```python
from build123d import *

# Parameters (mm, degrees)
SKETCH1_R           = 15
BOSS_EXTRUDE5_DEPTH = 40
SKETCH1_12_R        = 5
BOSS_EXTRUDE6_DEPTH = 8
SKETCH2_W           = 12
SKETCH2_H           = 18
CUT_EXTRUDE1_DEPTH  = 68


with BuildPart() as part:
    # Sketch1 → Boss-Extrude5 (new body)
    with BuildSketch(Plane.XY):
        with BuildLine():
            ThreePointArc((22.912878475, 10), (25, 0), (22.912878475, -10))
            ThreePointArc((22.912878475, -10), (0, -25), (-22.912878475, -10))
            ThreePointArc((-22.912878475, -10), (-25, 0), (-22.912878475, 10))
            ThreePointArc((-22.912878475, 10), (0, 25), (22.912878475, 10))
        make_face()
        Circle(SKETCH1_R, mode=Mode.SUBTRACT)
    extrude(amount=BOSS_EXTRUDE5_DEPTH)

    # Sketch1_12 → Boss-Extrude6 (add)
    with BuildSketch(Plane.XY):
        with BuildLine():
            Line((35, 10), (22.912878475, 10))
            ThreePointArc((22.912878475, 10), (25, 0), (22.912878475, -10))
            Line((22.912878475, -10), (35, -10))
            ThreePointArc((35, -10), (45, 0), (35, 10))
        make_face()
        with Locations((35, 0)):
            Circle(SKETCH1_12_R, mode=Mode.SUBTRACT)
        with BuildLine():
            ThreePointArc((-22.912878475, 10), (-25, 0), (-22.912878475, -10))
            Line((-22.912878475, -10), (-35, -10))
            ThreePointArc((-35, -10), (-45, 0), (-35, 10))
            Line((-35, 10), (-22.912878475, 10))
        make_face()
        with Locations((-35, 0)):
            Circle(SKETCH1_12_R, mode=Mode.SUBTRACT)
    extrude(amount=BOSS_EXTRUDE6_DEPTH)

    # Sketch2 → Cut-Extrude1 (cut)
    with BuildSketch(Plane(origin=(25, 0, 0), x_dir=(0, 0, -1), z_dir=(1, 0, 0))):
        with Locations((-34, 0)):
            Rectangle(SKETCH2_W, SKETCH2_H)
    extrude(amount=-CUT_EXTRUDE1_DEPTH, mode=Mode.SUBTRACT)


solid = part.part
```
Geometry: final body of the model. Coordinates: model frame, mm. A direction names the side the tool comes from. Round coordinates to 2 decimals unless told otherwise and drop trailing zeros. Loops run counter-clockwise (first coordinate to the right, second up) from the corner with the lowest first, then second, coordinate; pieces in that order, holes last. Notation, with made-up numbers: (-34.5, 39.5) -> (-22.5, 39.5) arc R10 cw to (-22.5, 43.5) -> close; hole circle Ø6 at (78.25, 75.25). An arc over 180 degrees is marked (long way). Write each question's results on one line, items separated by ' | '.
Item 1: Cut plane A-A on y = 0. Return the cut outline in (x, z), and give its area (3 significant figures).
Answers below:
outline: (-45, 0) -> (-40, 0) -> (-40, 8) -> (-45, 8) -> close; (-30, 0) -> (-15, 0) -> (-15, 28) -> (-25, 28) -> (-25, 8) -> (-30, 8) -> close; (15, 0) -> (30, 0) -> (30, 8) -> (25, 8) -> (25, 28) -> (15, 28) -> close; (40, 0) -> (45, 0) -> (45, 8) -> (40, 8) -> close | area: 720 mm²
Item 2: Cut plane D-D on y = 7.5. Return the cut outline in (x, z).
Answers below:
outline: (-41.61, 0) -> (-12.99, 0) -> (-12.99, 28) -> (-23.85, 28) -> (-23.85, 8) -> (-41.61, 8) -> close; (12.99, 0) -> (41.61, 0) -> (41.61, 8) -> (23.85, 8) -> (23.85, 28) -> (12.99, 28) -> close
Item 3: Set-up query: faces 5 (the face through (-29, -10, 4)), 6 (the face through (18, 9, 34)), 7 (the face through (29, -10, 4)). Return all of +Z, -Z, +X, -X, +Y, -Y with unobstructed straight access to the full face (end or side cutting, diameter ignored); none if empty.
Answers below:
face 5: +Z, -Z, -X, -Y | face 6: +Z, +X, -X | face 7: +Z, -Z, +X, -Y
Item 4: Cut plane C-C on z = 3.5. Return the cut outline in (x, y), and give its area (3 significant figures).
Answers below:
outline: (-35, -10) -> (-22.91, -10) arc R25 ccw to (22.91, -10) -> (35, -10) arc R10 ccw to (35, 10) -> (22.91, 10) arc R25 ccw to (-22.91, 10) -> (-35, 10) arc R10 ccw to start; hole circle Ø10 at (-35, 0); hole circle Ø30 at (0, 0); hole circle Ø10 at (35, 0) | area: 1,840 mm²
Item 5: Line query: probe 1 along X at (y, z) = (9, 8.5); probe 2 along Y at (x, z) = (35, 5.5); probe 3 along X at (y, z) = (4, 3). Output: solid intervals per line, ascending. Write a range as [from, to].
Answers below:
probe 1: x = [-23.32, -12], [12, 23.32] | probe 2: y = [-10, -5], [5, 10] | probe 3: x = [-44.17, -38], [-32, -14.46], [14.46, 32], [38, 44.17]
Item 6: Cut plane B-B on x = 0. Return the cut outline in (y, z).
Answers below:
outline: (-25, 0) -> (-15, 0) -> (-15, 40) -> (-25, 40) -> close; (15, 0) -> (25, 0) -> (25, 40) -> (15, 40) -> close
Item 7: Pull-direction query (Y, two-part tool) for faces 1 (the face through (-29, 10, 4)), 2 (the face through (0, -17, 40)), 3 (the face through (18, -9, 34)), 4 (the face through (-14.985, 0.66, 19.72)); classes: pulls with the +Y half, pulls with the -Y half, needs draft (parallel to the pull), parting line crosses it, or undercut.
Answers below:
face 1: pulls with the +Y half | face 2: needs draft | face 3: undercut | face 4: undercut
Item 8: Pin query (flat end, axial travel): pin 1 Ø1 at (x, z) = (-5, 25.5) entering from -Y; pin 2 Ø3.5 at (x, z) = (15, 36.5) entering from +Y; pin 3 Ø2.5 at (x, z) = (-27, 4.5) entering from -Y; pin 4 Ø1 at (x, y) = (13.5, -3.5) entering from +Z. Return the tip coordinate at first contact, or that it passes through.
Answers below:
pin 1: stops at y = -24.59 | pin 2: stops at y = 21.2 | pin 3: stops at y = -10 | pin 4: passes through
